```python
from build123d import *

# Parameters (mm, degrees)
SKETCH1_W           = 12.7
SKETCH1_H           = 76.2
BOSS_EXTRUDE1_DEPTH = 6.35
SKETCH2_R           = 2.383900133
CUT_EXTRUDE1_DEPTH  = 55.651998855
FILLET1_R           = 6.35


with BuildPart() as part:
    # Sketch1 → Boss-Extrude1 (new body)
    with BuildSketch(Plane.XY):
        with Locations((-0.022814859, 15.806453321)):
            Rectangle(SKETCH1_W, SKETCH1_H)
    extrude(amount=BOSS_EXTRUDE1_DEPTH)

    # Sketch2 → Cut-Extrude1 (cut, through all)
    with BuildSketch(Plane(origin=(0, 0, 0), x_dir=(-1, 0, 0), z_dir=(0, 0, -1))):
        Circle(SKETCH2_R)
    extrude(amount=-CUT_EXTRUDE1_DEPTH, mode=Mode.SUBTRACT)

    # Fillet1
    fillet1_edges = [part.edges().sort_by_distance(p)[0] for p in [
        (6.327185141, -22.293546679, 3.175),
        (-6.372814859, -22.293546679, 3.175),
        (6.327185141, 53.906453321, 3.175),
        (-6.372814859, 53.906453321, 3.175),
    ]]
    fillet(fillet1_edges, radius=FILLET1_R - 0.0001)  # a hair under: the kernel refuses the full size


solid = part.part
```
Can you work these out from the model? Positions are in its coordinate system, mm. Give positions to 0.01 mm unless a question says otherwise; leave off trailing zeros. Loops run counter-clockwise (first coordinate to the right, second up) from the corner with the lowest first, then second, coordinate; pieces in that order, holes last. Notation, with made-up numbers: M -29,-16 L 30,-16 A10 cw 30,-7 Z; hole C -30.5,-1.75 d3. An arc over 180 degrees is marked long. One line per item, written item: value.
(1) We'd pull the mould along X, two halves only. Please class faces 1 (the face through (0, 16, 6.35)), 2 (the face through (0.31, 2.364, 3.131)), 3 (the face through (4.418, 52.096, 3.219)): released by +X, released by -X, zero draft, split by the parting line, or undercut.
Returned:
face 1: zero draft
face 2: undercut
face 3: released by +X
(2) Suppose I cut it at C-C on x = 1. List the corners of the cut face in (y, z) for me.
Returned:
outline: M -22.21,0 L -2.16,0 L -2.16,6.35 L -22.21,6.35 Z; M 2.16,0 L 53.82,0 L 53.82,6.35 L 2.16,6.35 Z
(3) I need wall thicknesses on line 1 (Y direction, x = 0, z = 3.25); line 2 (Y direction, x = 1, z = 2.75); line 3 (Y direction, x = 4.5, z = 3). Which ranges of each line are inside material? Lowest first, please.
Returned:
line 1: -22.29 to -2.38, 2.38 to 53.91
line 2: -22.21 to -2.16, 2.16 to 53.82
line 3: -20.4 to 52.01
(4) Suppose I cut it at D-D on x = -5. List the corners of the cut face in (y, z) for me.
Returned:
outline: M -19.89,0 L 51.5,0 L 51.5,6.35 L -19.89,6.35 Z
(5) Suppose I cut it at A-A on y = 0. List the corners of the cut face in (x, z) for me.
Returned:
outline: M -6.37,0 L -2.38,0 L -2.38,6.35 L -6.37,6.35 Z; M 2.38,0 L 6.33,0 L 6.33,6.35 L 2.38,6.35 Z
(6) Will this pin go through, and if not, where does the flat tip stop? pin 1 (3 mm diameter, centred on x = -4.5, z = 3.5, fed in from -Y).
Returned:
pin 1: y = -21.55
